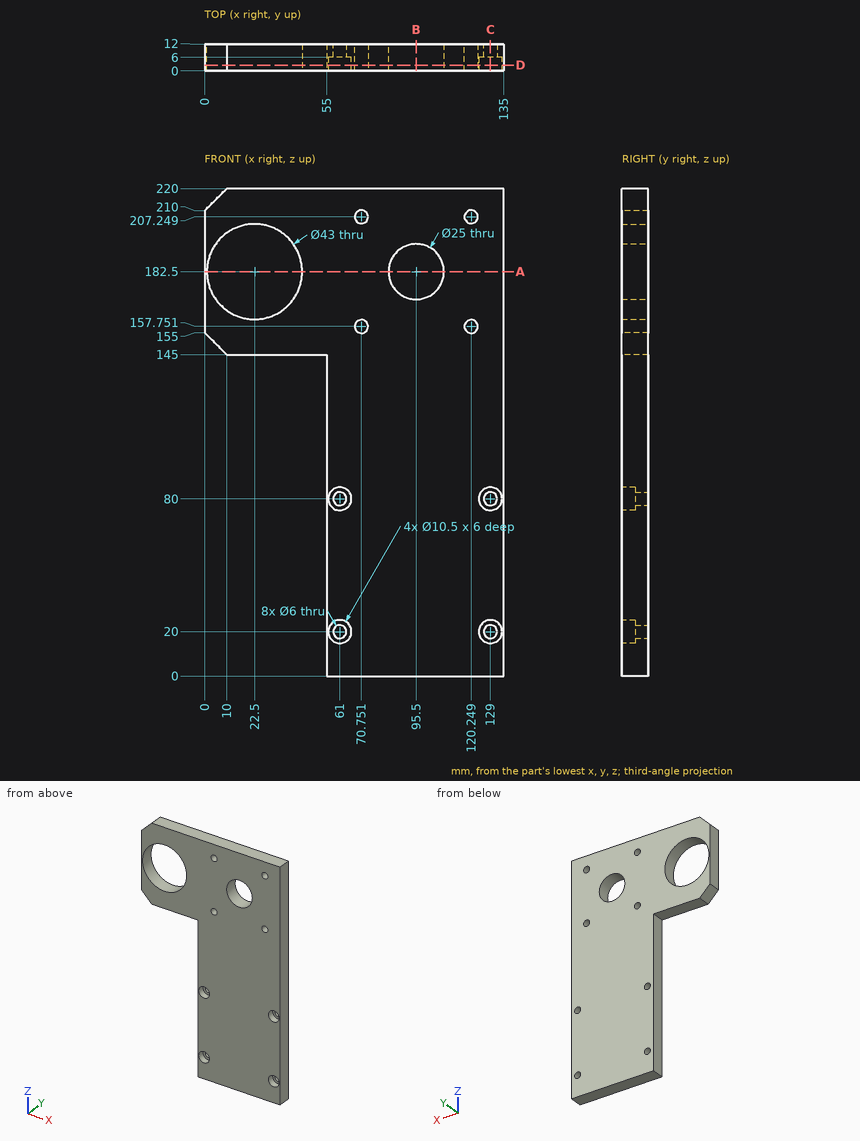
Drawing for the job (mm, zero at the part's lowest x, y, z). Coordinates: 2 decimals unless noted, no trailing zeros. Order: outer loops, then holes, each group sorted by start corner. A loop starts at its lowest first (then second) coordinate and runs counter-clockwise, first axis right, second up. Notation, with made-up numbers: (-31.75, 78) - (16.25, 78) arc R32 ccw to (16.25, 109) - close; hole circle Ø3 at (-37, 88.5). An arc over 180 degrees is marked (long way). Use a Markdown table: item, result. Add a question column.
(1) Flat gauge pins, fed straight in: pin 1 (5 mm diameter, centred on x = 128, z = 78.5, fed in from -Y); pin 2 (6 mm diameter, centred on y = 5, z = 59, fed in from -X). Where does each tip first touch, or does it go through?
(2) Saw through at C-C (x = 129). Give the cut face in (y, z).
(3) Saw through at A-A (z = 182.5). Give the cut face in (x, y).
(4) Saw through at B-B (x = 95.5). Give the cut face in (y, z), then the cut area to 3 significant figures.
(5) Saw through at D-D (y = 2.5). Count the separate pieces of the cut face and the enclosed holes in it, then the cut area to 3 significant figures.
(6) Drill centre lines: line 1 along Z through (x, y) = (128.5, 5.5); line 2 along Z through (x, y) = (61, 10.2); line 3 along X through (y, z) = (10, 208) (1 decimal). Where is each one in solid material? Low to high. Write a range as [from, to].
Solved:
| question | item | result |
|---|---|---|
| 1 | pin 1 | stops at y = 6 |
| 1 | pin 2 | stops at x = 55 |
| 2 | outline | (0, 0) - (12, 0) - (12, 17) - (6, 17) - (6, 14.75) - (0, 14.75) - close; (0, 25.25) - (6, 25.25) - (6, 23) - (12, 23) - (12, 77) - (6, 77) - (6, 74.75) - (0, 74.75) - close; (0, 85.25) - (6, 85.25) - (6, 83) - (12, 83) - (12, 220) - (0, 220) - close |
| 3 | outline | (0, 0) - (1, 0) - (1, 12) - (0, 12) - close; (44, 0) - (83, 0) - (83, 12) - (44, 12) - close; (108, 0) - (135, 0) - (135, 12) - (108, 12) - close |
| 4 | outline | (0, 0) - (12, 0) - (12, 170) - (0, 170) - close; (0, 195) - (12, 195) - (12, 220) - (0, 220) - close |
| 4 | area | 2,340 mm² |
| 5 | separate pieces | 1 |
| 5 | enclosed holes | 10 |
| 5 | area | 19,200 mm² |
| 6 | line 1 | z = [0, 14.77], [25.23, 74.77], [85.23, 220] |
| 6 | line 2 | z = [0, 17], [23, 77], [83, 220] |
| 6 | line 3 | x = [0, 67.8], [73.7, 117.3], [123.2, 135] |
